Build history of the part. All positions in model axes, mm. Round coordinates to 2 decimals unless told otherwise and drop trailing zeros. Write each loop counter-clockwise with the first axis right and the second up, starting at its lowest first coordinate (ties: lowest second). Pieces come first, ordered by that corner, then holes.
1) Saw through at A-A (y = -177.5). Write the cut outline in (x, z).
2) Saw through at C-C (z = -121). Write the cut outline in (x, y).
3) Saw through at D-D (y = -79.5). Write the cut outline in (x, z), plus the area to 3 significant figures.
4) Flat gauge pin, fed straight in: pin 1 (20.5 mm diameter, centred on x = 240.02, y = -167.6, fed in from +Z). Where does the tip first touch, or does it go through?
5) Saw through at B-B (x = 102.5). Write the cut outline in (y, z), plus the area to 3 significant figures.
6) Pull direction Y, two halves, no side cores. Call faces 1 (the flat face through (162, -231.098, -117)), 2 (the flat face through (68.572, -115, -117)), 3 (the flat face through (165, -2.498, -117)), 4 (the cylindrical face through (101.98, -97.64, -116.98)): +Y half, -Y half, draft (parallel to the pull), parting line (faces both ways), or undercut.
7) Wall check: probe 1 along Y at (x, z) = (106, -125.25); probe 2 along X at (y, z) = (-54, -123.25); probe 3 along X at (y, z) = (-158, -111.5). Give the ranges that are in metal, low to high.
Autodesk Inventor part; units mm, degrees
ref_plane "YZ Plane" through (0, 0, 0) normal (1, 0, 0) x (0, 1, 0)
ref_plane "XZ Plane" through (0, 0, 0) normal (0, 1, 0) x (-1, 0, 0)
ref_plane "XY Plane" through (0, 0, 0) normal (0, 0, 1) x (1, 0, 0)
ref_plane "Work Plane1" through (163.8219, -116.7983, -107.5891) normal (0, 0, -1) x (-1, 0, 0)
sketch "Sketch1" plane through (163.8219, -116.7983, -107.5891) normal (0, 0, -1) x (-1, 0, 0)
  line L0 (-95.25, 114.3) -> (95.25, 114.3)
  line L1 (95.25, 114.3) -> (95.25, -114.3)
  line L2 (95.25, -114.3) -> (-95.25, -114.3)
  line L3 (-95.25, -114.3) -> (-95.25, 114.3)
  line L4 (-95.25, 114.3) -> (95.25, -114.3) construction
  line L5 (95.25, 114.3) -> (-95.25, -114.3) construction
  arc A0 (44.45, 50.8) -> (25.4, 69.85) centre (25.4, 50.8) ccw construction
  line L6 (25.4, 69.85) -> (-25.4, 69.85) construction
  arc A1 (-25.4, 69.85) -> (-44.45, 50.8) centre (-25.4, 50.8) ccw construction
  line L7 (-44.45, 50.8) -> (-44.45, -50.8) construction
  arc A2 (-44.45, -50.8) -> (-25.4, -69.85) centre (-25.4, -50.8) ccw construction
  line L8 (-25.4, -69.85) -> (25.4, -69.85) construction
  arc A3 (25.4, -69.85) -> (44.45, -50.8) centre (25.4, -50.8) ccw construction
  line L9 (44.45, -50.8) -> (44.45, 50.8) construction
  line L10 (38.1, 50.8) -> (38.1, -50.8) construction
  arc A4 (25.4, -63.5) -> (38.1, -50.8) centre (25.4, -50.8) ccw construction
  line L11 (25.4, -63.5) -> (-25.4, -63.5) construction
  arc A5 (-38.1, -50.8) -> (-25.4, -63.5) centre (-25.4, -50.8) ccw construction
  line L12 (-38.1, -50.8) -> (-38.1, 50.8) construction
  arc A6 (-25.4, 63.5) -> (-38.1, 50.8) centre (-25.4, 50.8) ccw construction
  line L13 (-25.4, 63.5) -> (25.4, 63.5) construction
  arc A7 (38.1, 50.8) -> (25.4, 63.5) centre (25.4, 50.8) ccw construction
  circle A8 centre (-76.2, 63.5) radius 12.7
  circle A9 centre (-76.2, -50.8) radius 12.7
  circle A10 centre (63.5, 31.75) radius 12.7
  circle A11 centre (63.5, -31.75) radius 12.7
  point P0 (163.8219, 116.7983)
  point P1 (0, 0)
  point P2 (0, 63.5)
  point P3 (38.1, 0)
  dimension "d0" = 228.6
  dimension "d1" = 190.5
  dimension "d2" = 25.4
  dimension "d3" = 19.05
  dimension "d4" = 114.3
  dimension "d5" = 63.5
  dimension "d6" = 31.75
  dimension "d7" = 63.5
  dimension "d8" = 82.55
extrude "Extrusion1" add sketch "Sketch1" along normal blind 19.05
properties part number "class2" material "Iron, Ductile"
Evaluation:
1. outline: (68.57, -126.64) - (232.07, -126.64) - (232.07, -107.59) - (68.57, -107.59) - close; (247.97, -126.64) - (259.07, -126.64) - (259.07, -107.59) - (247.97, -107.59) - close
2. outline: (68.57, -231.1) - (259.07, -231.1) - (259.07, -2.5) - (68.57, -2.5) - close; hole circle Ø25.4 at (100.32, -148.55); hole circle Ø25.4 at (100.32, -85.05); hole circle Ø25.4 at (240.02, -167.6); hole circle Ø25.4 at (240.02, -53.3)
3. outline: (68.57, -126.64) - (88.9, -126.64) - (88.9, -107.59) - (68.57, -107.59) - close; (111.75, -126.64) - (259.07, -126.64) - (259.07, -107.59) - (111.75, -107.59) - close
3. area: 3,190 mm2
4. pin 1: passes through
5. outline: (-231.1, -126.64) - (-161.06, -126.64) - (-161.06, -107.59) - (-231.1, -107.59) - close; (-136.04, -126.64) - (-97.56, -126.64) - (-97.56, -107.59) - (-136.04, -107.59) - close; (-72.54, -126.64) - (-2.5, -126.64) - (-2.5, -107.59) - (-72.54, -107.59) - close
5. area: 3,400 mm2
6. face 1: -Y half
6. face 2: draft
6. face 3: +Y half
6. face 4: undercut
7. probe 1: y = -231.1 to -159.91, -137.19 to -96.41, -73.69 to -2.5
7. probe 2: x = 68.57 to 227.34, 252.7 to 259.07
7. probe 3: x = 68.57 to 91.84, 108.8 to 231.71, 248.34 to 259.07
